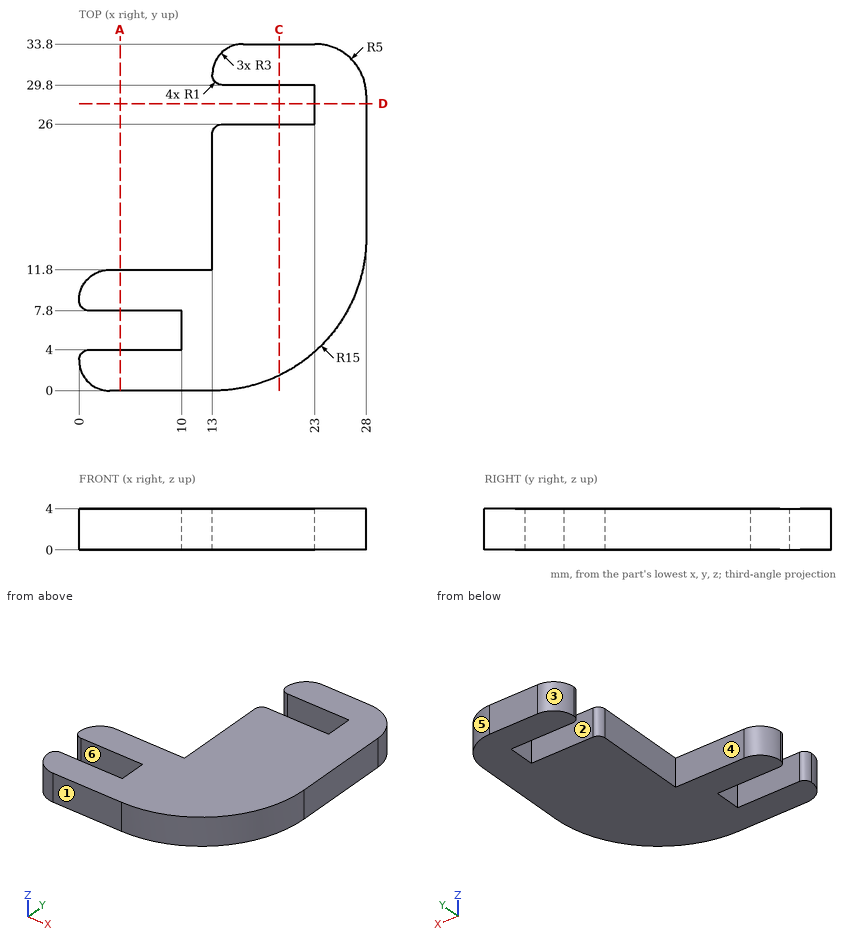
Can you work these out from the drawing? Everything is in mm from the part's minimum corner. A direction names the side the tool comes from. Coordinates: 2 decimals unless noted, no trailing zeros. Loops run counter-clockwise (first coordinate to the right, second up) from the corner with the lowest first, then second, coordinate; pieces in that order, holes last. Notation, with made-up numbers: (4.5, -37) - (40.5, -37) arc R13 ccw to (40.5, -31) - close; hole circle Ø3 at (61.5, -0.5). An arc over 180 degrees is marked (long way). Use a Markdown table: item, result.
Item 1: We'd pull the mould along Y, two halves only. Please class the marked faces 1, 2 and 3: released by +Y, released by -Y, zero draft, split by the parting line, or undercut.
Numbers:
| item | result |
|---|---|
| face 1 | released by -Y |
| face 2 | undercut |
| face 3 | released by +Y |
Item 2: I want a section at D-D on y = 28. Please give me the cut outline in (x, z).
Numbers:
| item | result |
|---|---|
| outline | (23, 0) - (28, 0) - (28, 4) - (23, 4) - close |
Item 3: Will these pins go through, and if not, where does the flat tip stop? pin 1 (2 mm diameter, centred on x = 19.5, z = 3, fed in from -Y); pin 2 (1.1 mm diameter, centred on y = 6.5, z = 2, fed in from -X); pin 3 (2 mm diameter, centred on y = 19, z = 3, fed in from -X).
Numbers:
| item | result |
|---|---|
| pin 1 | stops at y = 1.04 |
| pin 2 | stops at x = 10 |
| pin 3 | stops at x = 13 |
Item 4: For the marked faces 4, 5 and 6, which set-ups out of +Z, -Z, +X, -X, +Y, -Y let a thin tool reach every point of the face, with its end or its side?
Numbers:
| item | result |
|---|---|
| face 4 | +Z, -Z, -X, +Y |
| face 5 | +Z, -Z, +X, +Y |
| face 6 | +Z, -Z, -X |
Item 5: If I drill on probe 1 along Y at (x, z) = (9.5, 1.4); probe 2 along X at (y, z) = (19, 0.85); probe 3 along X at (y, z) = (26.5, 3.1), over which ranges is the centre line in solid material (lowest first)? Write a range as from..to.
Numbers:
| item | result |
|---|---|
| probe 1 | y = 0..4, 7.8..11.8 |
| probe 2 | x = 13..28 |
| probe 3 | x = 23..28 |
Item 6: I want a section at C-C on x = 19.5. Please give me the cut outline in (y, z).
Numbers:
| item | result |
|---|---|
| outline | (1.48, 0) - (26, 0) - (26, 4) - (1.48, 4) - close; (29.8, 0) - (33.8, 0) - (33.8, 4) - (29.8, 4) - close |
Item 7: I want a section at A-A on x = 4. Please give me the cut outline in (y, z).
Numbers:
| item | result |
|---|---|
| outline | (0, 0) - (4, 0) - (4, 4) - (0, 4) - close; (7.8, 0) - (11.8, 0) - (11.8, 4) - (7.8, 4) - close |
